For this review, take the finished solid that the model builds, in its own axes (mm). A direction names the side the tool comes from. Coordinates: 2 decimals unless noted, no trailing zeros. Order: outer loops, then holes, each group sorted by start corner. A loop starts at its lowest first (then second) coordinate and runs counter-clockwise, first axis right, second up. Notation, with made-up numbers: (84.5, -8) -> (98.5, -8) arc R28 ccw to (98.5, 21) -> close; hole circle Ø9 at (40, 58.25). An arc over 180 degrees is marked (long way). Return JSON: item names as keys, results as strings. Group by question number.
Item 1: Take a section at D-D (y = 48). Write out the cut boundary in (x, z), then the cut area to 3 significant figures.
Item 2: Take a section at B-B (x = 45.25). Count the separate pieces of the cut face and the enclosed holes in it, then the cut area to 3 significant figures.
Item 3: Insertion check: pin 1 (2.5 mm diameter, centred on x = 38.5, y = 37.5, fed in from +Z); pin 2 (3 mm diameter, centred on x = 43.5, y = 71.5, fed in from -Z); pin 3 (4 mm diameter, centred on x = 38.5, y = 72, fed in from -Z). Each pin has a flat end and moves straight along its axis. Give the tip position at first contact, or say it passes through.
Item 4: Take a section at C-C (z = 7). Write out the cut boundary in (x, y), then the cut area to 3 significant figures.
Item 5: For line 1 along Y through (x, z) = (36.7, 7); line 2 along Y through (x, z) = (44.5, 25.75); line 3 along Y through (x, z) = (44.5, 12.75), list the stretches that pass through material, from the lowest coordinate up.
Item 6: Machinability: for faces 5 (the flat face through (37, 58.251, 7)), 6 (the cylindrical face through (43.673, 49.954, 9.395)), 7 (the cylindrical face through (41.278, 39.328, 13.599)), which of the approach directions +Z, -Z, +X, -X, +Y, -Y give a long, thin tool a straight path to every point of the face, cutting with its end or side? Answer none if there is none.
Item 7: Draft analysis for pull direction Z (two halves, no side actions). For faces 1 (the flat face through (40, 58, 18)), 2 (the flat face through (41, 34, 6)), 3 (the cylindrical face through (43.673, 32.008, 10.247)), 4 (the flat face through (36, 42, 0)), state which applies: +Z half, -Z half, draft (parallel to the pull), parting line (faces both ways), or undercut.
Item 8: Take a section at A-A (z = 19.25). Write out the cut boundary in (x, y), then the cut area to 3 significant figures.
Autodesk Inventor part; units mm, degrees
ref_plane "YZ Plane" through (0, 0, 0) normal (1, 0, 0) x (0, 1, 0)
ref_plane "XZ Plane" through (0, 0, 0) normal (0, 1, 0) x (-1, 0, 0)
ref_plane "XY Plane" through (0, 0, 0) normal (0, 0, 1) x (1, 0, 0)
ref_plane "Arbeitsebene2" through (35, 26.0506, 0) normal (1, 0, 0) x (0, 0, -1)
sketch "Skizze6" plane through (35, 26.0506, 0) normal (1, 0, 0) x (0, 0, -1)
  line L0 (-14, 32.2) -> (-14, 0)
  line L1 (0, 0) -> (-14, 0)
  line L2 (0, 32.2) -> (0, 0)
  line L3 (0, 32.2) -> (-14, 32.2)
  line L4 (-8.5, 27.35) -> (0, 27.35)
  line L5 (-8.5, 24.85) -> (0, 24.85)
  line L6 (-8.5, 7.35) -> (0, 7.35)
  line L7 (-8.5, 4.85) -> (0, 4.85)
  circle A0 centre (-7, 26.1) radius 1.6
  circle A1 centre (-7, 6.1) radius 1.6
  point P0 (0, -26.0506)
  dimension "d40" = 3.2
  dimension "d41" = 3.2
  dimension "d42" = 1.25
  dimension "d43" = 1.25
  dimension "d44" = 7
  dimension "d45" = 7
extrude "Extrusion6" add sketch "Skizze6" along normal blind 5 contours L3 L2 L4 A0 L5 L6 A1 L7 L1 L0 | L2 L5 A0 L4 | L7 A1 L6 L2
sketch "Skizze7" plane through (40, 26.0506, 0) normal (1, 0, 0) x (0, 0, -1)
  line L0 (0, 32.2) -> (-14, 32.2)
  line L1 (-14, 32.2) -> (-14, 0)
  line L2 (-14, 0) -> (0, 0)
  line L3 (0, 0) -> (0, 32.2)
  circle A0 centre (-7, 26.1) radius 1.6
  circle A1 centre (-7, 6.1) radius 1.6
  line L4 (-58.75, 26.0265) -> (-58.75, 86.0265)
  line L5 (0, 32.2) -> (-27.8, 32.2)
  line L6 (-27.8, 32.2) -> (-27.8, 0)
  line L7 (-27.8, 0) -> (0, 0)
  line L8 (0, 0) -> (0, 32.2)
  line L9 (0, 32.2) -> (-14, 32.2)
  line L10 (0, 32.2) -> (-27.8, 32.2)
  line L11 (-27.8, 32.2) -> (-27.8, 52.2)
  line L12 (-27.8, 52.2) -> (0, 52.2)
  line L13 (0, 52.2) -> (0, 32.2)
  point P0 (0, -26.0506)
  point P1 (-14, 0)
  point P2 (-14, 32.2)
  dimension "d48" = 27.8
  dimension "d51" = 20
extrude "Extrusion7" add sketch "Skizze7" along normal blind 8
sketch "Skizze8" plane through (35, 26.0506, 0) normal (0, 0, -1) x (-1, 0, 0)
  line L0 (-13, 24.5) -> (0, 24.5)
  line L1 (-13, 27.7) -> (0, 27.7)
  line L2 (-13, 7.7) -> (0, 7.7)
  line L3 (-13, 4.5) -> (0, 4.5)
  line L4 (0, 0) -> (0, 32.2)
  line L5 (0, 32.2) -> (-5, 32.2)
  line L6 (-5, 32.2) -> (-5, 52.2)
  line L7 (-5, 52.2) -> (-13, 52.2)
  line L8 (-13, 0) -> (-13, 52.2)
  line L9 (0, 0) -> (-13, 0)
  circle A0 centre (-9.5, 39.8052) radius 1.6 construction
  circle A1 centre (-9.5, 13.7) radius 1.4 construction
  circle A2 centre (-9.5, 29.7) radius 1.4 construction
  circle A3 centre (-9.5, 45.7) radius 1.4 construction
  point P0 (35, -26.0506)
  dimension "d52" = 2.8
  dimension "d53" = 3.5
  dimension "d54" = 6
  dimension "d55" = 2.8
  dimension "d56" = 16
  dimension "d57" = 2.8
  dimension "d58" = 16
hole "Bohrung1" at (44.5, 39.7506, 0) at (44.5, 55.7506, 0) at (44.5, 71.7506, 0) direction (0, 0, 1) diameter 3.2 end through all counterbore diameter 6.5 counterbore depth 20
chamfer "Fase4" distance 10 angle 45 1 edges at (48, 52.1506, 0)
sketch "Skizze9" plane through (48, 26.0506, 0) normal (1, 0, 0) x (0, 0, -1)
  circle A0 centre (-7, 6.1) radius 1.6
  arc A1 (-8.3185, 27.0064) -> (-5.4844, 26.6128) centre (-7, 26.1) ccw
  point P0 (0, -26.0506)
hole "Bohrung2" at (48, 32.1506, 7) at (48, 52.1506, 7) direction (-1, 0, 0) diameter 3.2 end through all counterbore diameter 6.5 counterbore depth 7
properties part number "30_XYTable_Aliexpress_Translatorarm_y"
Findings below:
{
 "1": {"outline": "(35, 0) -> (38, 0) -> (48, 10) -> (48, 27.8) -> (40, 27.8) -> (40, 14) -> (35, 14) -> close", "area": "242 mm2"},
 "2": {"separate pieces": "4", "enclosed holes": "0", "area": "741 mm2"},
 "3": {"pin 1": "stops at z = 14", "pin 2": "stops at z = 20", "pin 3": "stops at z = 2"},
 "4": {"outline": "(35, 26.05) -> (45, 26.05) -> (45, 28.9) -> (41, 28.9) -> (41, 30.55) -> (35, 30.55) -> close; (35, 33.75) -> (41, 33.75) -> (41, 35.4) -> (45, 35.4) -> (45, 36.54) arc R3.25 cw (long way) to (45, 42.96) -> (45, 48.9) -> (41, 48.9) -> (41, 50.55) -> (35, 50.55) -> close; (35, 53.75) -> (41, 53.75) -> (41, 55.4) -> (41.27, 55.4) arc R3.25 cw to (45, 58.96) -> (45, 68.54) arc R3.25 cw (long way) to (45, 74.96) -> (45, 78.25) -> (40, 78.25) -> (40, 58.25) -> (35, 58.25) -> close", "area": "281 mm2"},
 "5": {"line 1": "y = 26.05 to 30.55, 33.75 to 50.55, 53.75 to 58.25", "line 2": "y = 26.05 to 38.15, 41.35 to 54.15, 57.35 to 70.15, 73.35 to 78.25", "line 3": "y = 26.05 to 36.5, 43 to 52.5, 59 to 68.5, 75 to 78.25"},
 "6": {"face 5": "+Z, -Z, -X, +Y", "face 6": "+X", "face 7": "-Z"},
 "7": {"face 1": "draft", "face 2": "undercut", "face 3": "undercut", "face 4": "-Z half"},
 "8": {"outline": "(40, 26.05) -> (48, 26.05) -> (48, 78.25) -> (40, 78.25) -> close; hole circle Ø6.5 at (44.5, 39.75); hole circle Ø6.5 at (44.5, 55.75); hole circle Ø6.5 at (44.5, 71.75)", "area": "318 mm2"}
}
